The listing builds one solid part. Answer for the finished solid, in the listing's coordinates (mm). A direction names the side the tool comes from. Give positions to 0.01 mm unless a question says otherwise; leave off trailing zeros. Loops run counter-clockwise (first coordinate to the right, second up) from the corner with the lowest first, then second, coordinate; pieces in that order, holes last. Notation, with made-up numbers: (-1, 85) - (27, 85) arc R9 cw to (27, 97) - close; hole circle Ø10 at (-21.75, 13). An arc over 180 degrees is marked (long way). Write each question's results on one line, items separated by ' | '.
from build123d import *

# Parameters (mm, degrees)
CROQUIS1_R              = 1.8
SALIENTE_EXTRUIR1_DEPTH = 1.7
CROQUIS2_W              = 1.7
CROQUIS2_H              = 40
SALIENTE_EXTRUIR2_DEPTH = 60
CORTAR_EXTRUIR1_DEPTH   = 10
CROQUIS3_4_R            = 1.5
CORTAR_EXTRUIR2_DEPTH   = 10


with BuildPart() as part:
    # Croquis1 → Saliente-Extruir1 (new body)
    with BuildSketch(Plane.XY):
        Polygon((0, 0), (8, 0), (41, 0), (41, 40), (8, 40), (0, 40), align=None)
        with Locations((8, 5)):
            Circle(CROQUIS1_R, mode=Mode.SUBTRACT)
        with Locations((8, 35)):
            Circle(CROQUIS1_R, mode=Mode.SUBTRACT)
        with Locations((32, 5)):
            Circle(CROQUIS1_R, mode=Mode.SUBTRACT)
        with Locations((32, 35)):
            Circle(CROQUIS1_R, mode=Mode.SUBTRACT)
    extrude(amount=SALIENTE_EXTRUIR1_DEPTH)

    # Croquis2 → Saliente-Extruir2 (add)
    with BuildSketch(Plane.XY.offset(1.7)):
        with Locations((40.15, 20)):
            Rectangle(CROQUIS2_W, CROQUIS2_H)
    extrude(amount=SALIENTE_EXTRUIR2_DEPTH)

    # Croquis3 → Cortar-Extruir1 (cut)
    with BuildSketch(Plane.ZY.offset(-39.3)):
        with BuildLine():
            Line((61.7, 40), (28.7, 40))
            ThreePointArc((28.7, 40), (48.7, 20), (28.7, 0))
            Line((28.7, 0), (61.7, 0))
            Line((61.7, 0), (61.7, 40))
        make_face()
        with BuildLine():
            Line((21.7, 13.5), (35.7, 13.5))
            ThreePointArc((35.7, 13.5), (42.2, 20), (35.7, 26.5))
            Line((35.7, 26.5), (21.7, 26.5))
            ThreePointArc((21.7, 26.5), (15.2, 20), (21.7, 13.5))
        make_face()
    extrude(amount=-CORTAR_EXTRUIR1_DEPTH, mode=Mode.SUBTRACT)

    # Croquis3<4> → Cortar-Extruir2 (cut)
    with BuildSketch(Plane.ZY.offset(-39.3)):
        with Locations((15.406510052, 27.675)):
            Circle(CROQUIS3_4_R)
        with Locations((28.7, 35.35)):
            Circle(CROQUIS3_4_R)
        with Locations((41.993489948, 27.675)):
            Circle(CROQUIS3_4_R)
        with Locations((41.993489948, 12.325)):
            Circle(CROQUIS3_4_R)
        with Locations((28.7, 4.65)):
            Circle(CROQUIS3_4_R)
        with Locations((15.406510052, 12.325)):
            Circle(CROQUIS3_4_R)
    extrude(amount=-CORTAR_EXTRUIR2_DEPTH, mode=Mode.SUBTRACT)


solid = part.part
Item 1: A cutting plane is placed at C-C, the plane z = 25. Determine the outline of the cut face in (x, y), plus the area to 3 significant figures.
Values found:
outline: (39.3, 0) - (41, 0) - (41, 13.5) - (39.3, 13.5) - close; (39.3, 26.5) - (41, 26.5) - (41, 40) - (39.3, 40) - close | area: 45.9 mm²
Item 2: Find the intervals of material crossed by line 1 along Y through (x, z) = (8, 0.8); line 2 along Z through (x, y) = (28.5, 16); line 3 along X through (y, z) = (34, 7), in increasing order. Write a range as [from, to].
Values found:
line 1: y = [0, 3.2], [6.8, 33.2], [36.8, 40] | line 2: z = [0, 1.7] | line 3: x = [39.3, 41]
Item 3: For a pull along X with two mould halves and no side action, classify faces 1 (the face through (0, 20, 1)), 2 (the face through (26.5, 0, 1.5)), 3 (the face through (7.766, 36.785, 0.838)) as released by +X, released by -X, zero draft, split by the parting line, or undercut.
Values found:
face 1: released by -X | face 2: zero draft | face 3: undercut
Item 4: A cutting plane is placed at B-B, the plane y = 20. Determine the outline of the cut face in (x, z).
Values found:
outline: (0, 0) - (41, 0) - (41, 15.2) - (39.3, 15.2) - (39.3, 1.7) - (0, 1.7) - close; (39.3, 42.2) - (41, 42.2) - (41, 48.7) - (39.3, 48.7) - close
Item 5: For faces 4 (the face through (40.1, 20.1, 15.2)), 5 (the face through (33.663, 4.311, 0.838)), 6 (the face through (19, 20, 1.7)), determine the directions among +Z, -Z, +X, -X, +Y, -Y from which every point of the face is accessible in a straight line to the end or side of a thin tool.
Values found:
face 4: +X, -X | face 5: +Z, -Z | face 6: +Z, -X, +Y, -Y
Item 6: Flat-ended cylindrical pins translate along their axes: P1, Ø0.5, axis at x = 40, z = 31, coming from the -Y side; P2, Ø19.5, axis at x = 10.5, y = 20.5, coming from the +Z side; P3, Ø5, axis at y = 13, z = 24, coming from the -X side. Find the tip coordinate at first contact, or state that the pin passes through.
Values found:
P1: stops at y = 0.11 | P2: stops at z = 1.7 | P3: stops at x = 39.3
Item 7: A cutting plane is placed at D-D, the plane x = 22.5. Determine the outline of the cut face in (y, z).
Values found:
outline: (0, 0) - (40, 0) - (40, 1.7) - (0, 1.7) - close
Item 8: A cutting plane is placed at A-A, the plane x = 32. Determine the outline of the cut face in (y, z), plus the area to 3 significant figures.
Values found:
outline: (0, 0) - (3.2, 0) - (3.2, 1.7) - (0, 1.7) - close; (6.8, 0) - (33.2, 0) - (33.2, 1.7) - (6.8, 1.7) - close; (36.8, 0) - (40, 0) - (40, 1.7) - (36.8, 1.7) - close | area: 55.8 mm²
